from build123d import *

# Parameters (mm, degrees)
SKETCH_1_R      = 10.5
EXTRUDE_1_DEPTH = 21
SKETCH_2_R      = 8
EXTRUDE_2_DEPTH = 4
FILLET_1_R      = 2
SKETCH_3_R      = 1
EXTRUDE_3_DEPTH = 10


with BuildPart() as part:
    # 草圖1 → 填料-伸長1 (new body)
    with BuildSketch(Plane(origin=(0, 0, 0), x_dir=(1, 0, 0), z_dir=(0, 1, 0))):
        with Locations(Location((0, 0, 0), (0, 0, 90))):
            Circle(SKETCH_1_R)
    extrude(amount=EXTRUDE_1_DEPTH)

    # 草圖2 → 填料-伸長2 (add)
    with BuildSketch(Plane(origin=(0, 21, 0), x_dir=(1, 0, 0), z_dir=(0, 1, 0))):
        with Locations(Location((0, 0, 0), (0, 0, 270))):
            Circle(SKETCH_2_R)
    extrude(amount=EXTRUDE_2_DEPTH)

    # 圓角1
    fillet_1_edges = [part.edges().sort_by_distance(p)[0] for p in [
        (0, 25, -8),
    ]]
    fillet(fillet_1_edges, radius=FILLET_1_R)

    # 草圖3 → 填料-伸長3 (add)
    with BuildSketch(Plane(origin=(0, 25, 0), x_dir=(1, 0, 0), z_dir=(0, 1, 0))):
        with Locations(Location((0, 0, 0), (0, 0, 270))):
            Circle(SKETCH_3_R)
    extrude(amount=EXTRUDE_3_DEPTH)


solid = part.part
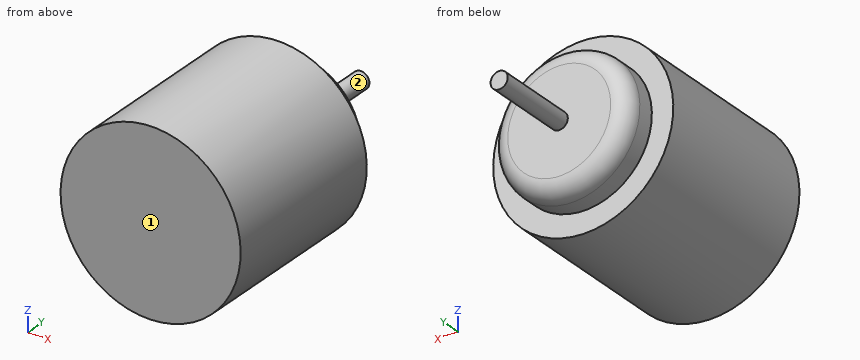
Could you check a few things on this model? Use its own coordinates, in mm. Face numbers are marked on the shaded views. A direction names the side the tool comes from. Give positions to 0.01 mm unless a question says otherwise; leave off trailing zeros. Write each loop counter-clockwise with the first axis right and the second up, starting at its lowest first coordinate (ties: lowest second). Pieces come first, ordered by that corner, then holes. Notation, with made-up numbers: (-23.75, 81) -> (6.25, 81) arc R26 ccw to (6.25, 98) -> close; hole circle Ø11 at (28.25, -0.5). An arc over 180 degrees is marked (long way). Write each question's results on one line, items separated by ' | '. Start each with the question number.
Q1. Suppose I cut it at B-B, the plane z = 0. List the corners of the cut face in (x, y) for me.
Q2. I'm going to push flat-ended pins straight in: pin 1 Ø1 at (y, z) = (13.5, 7.5) entering from +X; pin 2 Ø4 at (x, z) = (-4.5, -5) entering from +Y; pin 3 Ø1.5 at (x, y) = (-1, 16.5) entering from -Z. Where does each tip first touch, or does it pass through?
Q3. I need wall thicknesses on probe 1 along Y at (x, z) = (-8.5, -1.25); probe 2 along Y at (x, z) = (-3.75, -4); probe 3 along X at (y, z) = (11, 0). Which ranges of each line are inside material? Lowest first, please.
Q4. Suppose I cut it at D-D, the plane y = 26. List the corners of the cut face in (x, z) for me.
Q5. Suppose I cut it at C-C, the plane y = 22.5. List the corners of the cut face in (x, z) for me.
Q6. Suppose I cut it at A-A, the plane x = 0. List the corners of the cut face in (y, z) for me, and give its area (3 significant figures).
Q7. Which directions (+Z, -Z, +X, -X, +Y, -Y) give clear straight access to the entire face, cutting with the end or side of a thin tool? Please do the marked faces 1 and 2.
Outcome:
1) outline: (-10.5, 0) -> (10.5, 0) -> (10.5, 21) -> (8, 21) -> (8, 23) arc R2 ccw to (6, 25) -> (1, 25) -> (1, 35) -> (-1, 35) -> (-1, 25) -> (-6, 25) arc R2 ccw to (-8, 23) -> (-8, 21) -> (-10.5, 21) -> close
2) pin 1: x = 7.83 | pin 2: y = 25 | pin 3: z = -10.5
3) probe 1: 0 to 21 | probe 2: 0 to 25 | probe 3: -10.5 to 10.5
4) outline: circle Ø2 at (0, 0)
5) outline: circle Ø16 at (0, 0)
6) outline: (0, -10.5) -> (21, -10.5) -> (21, -8) -> (23, -8) arc R2 ccw to (25, -6) -> (25, -1) -> (35, -1) -> (35, 1) -> (25, 1) -> (25, 6) arc R2 ccw to (23, 8) -> (21, 8) -> (21, 10.5) -> (0, 10.5) -> close | area: 523 mm2
7) face 1: +Z, -Z, +X, -X, -Y | face 2: +Y
